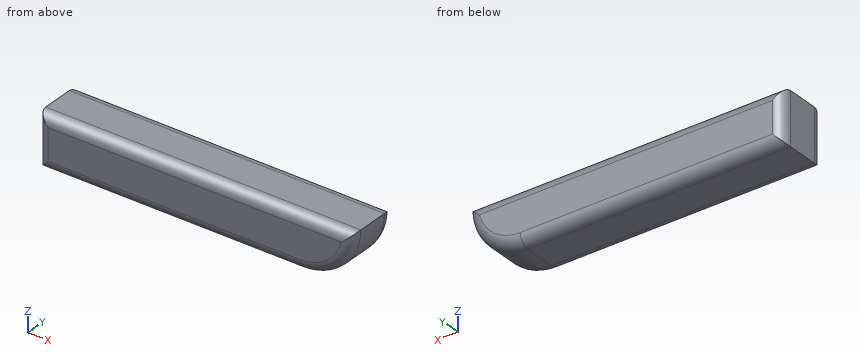
from build123d import *

# Parameters (mm, degrees)
F0_W     = 127
F0_H     = 25.4
F1_DEPTH = 25.4
F2_R     = 5.08


# Not quite as in the source:
# - a feature names something its author has since deleted; it is built from what else it names


with BuildPart() as f1:
    # F0 (on Front) → F1 (new body)
    with BuildSketch(Plane.XZ):
        with Locations((-12.2346525788, -22.7242771864)):
            Rectangle(F0_W, F0_H)
        with BuildLine():
            Line((76.6653474212, -10.0242771864), (51.2653474212, -10.0242771864))
            Line((51.2653474212, -10.0242771864), (51.2653474212, -35.4242771864))
            ThreePointArc((51.2653474212, -35.4242771864), (69.2258596633, -27.9847894285), (76.6653474212, -10.0242771864))
        make_face()
    extrude(amount=F1_DEPTH)

    # F2
    f2_edges = [f1.edges().sort_by_distance(p)[0] for p in [
        (-75.734653, -25.4, -22.724277),
        (-12.234653, -25.4, -35.424277),
        (69.22586, -25.4, -27.984789),
        (0.465347, -25.4, -10.024277),
        (-75.734653, 0, -22.724277),
        (-12.234653, 0, -35.424277),
        (69.22586, 0, -27.984789),
        (0.465347, 0, -10.024277),
    ]]
    fillet(f2_edges, radius=F2_R)


solid = f1.part
Here's how the part is built. I have some questions about the finished solid (model axes, mm). Coordinates: 2 decimals unless noted, no trailing zeros. Order: outer loops, then holes, each group sorted by start corner. A loop starts at its lowest first (then second) coordinate and runs counter-clockwise, first axis right, second up. Notation, with made-up numbers: (83.25, -15) - (89.25, -15) arc R6 cw to (89.25, -5) - close; hole circle Ø2 at (19.5, 86). An arc over 180 degrees is marked (long way). Use CSV: the item, a comma, the result in double quotes. Start each with the question number.
1. Please list where these lines run through material, in increasing order: line 1 (Y direction, x = -55, z = -15); line 2 (X direction, y = -22, z = -28.75); line 3 (X direction, y = -22.75, z = -10.75). Write a range as from..to.
2. Suppose I cut it at A-A on x = -42.5. List the corners of the cut face in (y, z) for me.
3. I'm going to push flat-ended pins straight in: pin 1 (1.5 mm diameter, centred on y = -22, z = -31.5, fed in from +X); pin 2 (10 mm diameter, centred on x = -51, z = -32, fed in from +Y); pin 3 (1 mm diameter, centred on y = -5, z = -27, fed in from +X). Where does each tip first touch, or does it pass through?
4. Suppose I cut it at B-B on y = -10.75. List the corners of the cut face in (x, z) for me, then the cut area to 3 significant figures.
Output:
1,line 1,"y = -25.4..0"
1,line 2,"x = -75.45..68"
1,line 3,"x = -75.12..76.04"
2,outline,"(-25.4, -30.34) arc R5.08 ccw to (-20.32, -35.42) - (-5.08, -35.42) arc R5.08 ccw to (0, -30.34) - (0, -15.1) arc R5.08 ccw to (-5.08, -10.02) - (-20.32, -10.02) arc R5.08 ccw to (-25.4, -15.1) - close"
3,pin 1,"stops at x = 65.53"
3,pin 2,"stops at y = 0"
3,pin 3,"stops at x = 70.6"
4,outline,"(-75.73, -35.42) - (51.27, -35.42) arc R25.4 ccw to (76.67, -10.02) - (-75.73, -10.02) - close"
4,area,"3,730 mm2"
